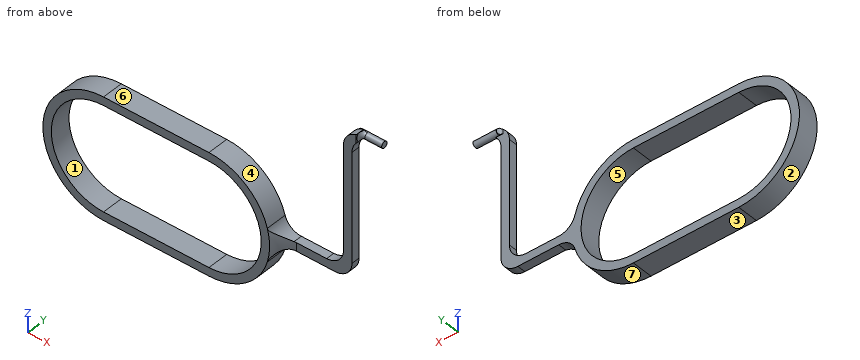
from build123d import *

# Parameters (mm, degrees)
BOSS_EXTRUDE1_DEPTH      = 5
BOSS_EXTRUDE2_START      = 2
SKETCH2_W                = 2
SKETCH2_H                = 2
SKETCH2_H_2              = 30.5
SKETCH2_W_2              = 1
BOSS_EXTRUDE2_DEPTH      = 2
FILLET1_R                = 4
BOSS_EXTRUDE3_DEPTH      = 5
BOSS_EXTRUDE3_DEPTH_BACK = 0.5
SKETCH3_R                = 0.75
FILLET2_R                = 1


with BuildPart() as part:
    # Sketch1 → Boss-Extrude1 (new body)
    with BuildSketch(Plane(origin=(0, 0, 0), x_dir=(1, 0, 0), z_dir=(0, 1, 0))):
        with BuildLine():
            Line((0, 14.4), (25, 14.4))
            ThreePointArc((25, 14.4), (39.4, 0), (25, -14.4))
            Line((25, -14.4), (0, -14.4))
            ThreePointArc((0, -14.4), (-14.4, 0), (0, 14.4))
        make_face()
        with BuildLine():
            Line((0, 12.4), (25, 12.4))
            ThreePointArc((25, 12.4), (37.4, 0), (25, -12.4))
            Line((25, -12.4), (0, -12.4))
            ThreePointArc((0, -12.4), (-12.4, 0), (0, 12.4))
        make_face(mode=Mode.SUBTRACT)
    extrude(amount=BOSS_EXTRUDE1_DEPTH)

    # Sketch2 → Boss-Extrude2 (add)
    with BuildSketch(Plane.XZ.offset(-5).offset(BOSS_EXTRUDE2_START)):
        with BuildLine():
            Line((39.365235814, -1), (54.4, -1))
            Line((54.4, -1), (54.4, 1))
            Line((54.4, 1), (39.365235814, 1))
            ThreePointArc((39.365235814, 1), (39.4, 0), (39.365235814, -1))
        make_face()
        with BuildLine():
            Line((37.4, -1), (39.365235814, -1))
            ThreePointArc((39.365235814, -1), (39.4, 0), (39.365235814, 1))
            Line((39.365235814, 1), (37.4, 1))
            Line((37.4, 1), (37.4, -1))
        make_face()
        with Locations((55.4, 0)):
            Rectangle(SKETCH2_W, SKETCH2_H)
        with Locations((55.4, 16.25)):
            Rectangle(SKETCH2_W, SKETCH2_H_2)
        with Locations((55.4, 32.5)):
            Rectangle(SKETCH2_W, SKETCH2_H)
        with Locations((56.9, 32.5)):
            Rectangle(SKETCH2_W_2, SKETCH2_H)
    extrude(amount=-BOSS_EXTRUDE2_DEPTH)

    # Fillet1
    # the kernel refuses this fillet: 4 mm, written as the material it adds along each edge
    with BuildSketch(Plane(origin=(25, 3, 0), x_dir=(0.7371891614816782, 0, -0.6756864214959037), z_dir=(-0.6756864214959037, 0, -0.7371891614816782))) as fillet1_piece_1_section:
        with BuildLine():
            CenterArc((18.272983346, 4), FILLET1_R, 194.477512186, 75.522487814)
            Line((18.272983346, 0), (18.272983346, -0.08))
            Line((18.272983346, -0.08), (14.4, -0.08))
            Line((14.4, -0.08), (14.32, 0))
            ThreePointArc((14.32, 0), (14.32, 1.5), (14.322540333, 2.98))
            Line((14.322540333, 2.98), (14.4, 3))
        make_face()
    fillet1_piece_1 = revolve(axis=Axis((25, 3, 0), (0, -1, 0)), revolution_arc=85.014954966, mode=Mode.PRIVATE)
    fillet1_piece_1 = split(fillet1_piece_1, bisect_by=Plane(origin=(40.301586348, 2.241602013, 1), z_dir=(0, 0, -1)), keep=Keep.TOP, mode=Mode.PRIVATE)
    fillet1_piece_1 = split(fillet1_piece_1, bisect_by=Plane(origin=(40.301586348, 2.241602013, -1), z_dir=(0, 0, 1)), keep=Keep.TOP, mode=Mode.PRIVATE)
    add(fillet1_piece_1)
    with BuildSketch(Plane(origin=(39.365235814, 5, 1), x_dir=(-0.17149804582148107, 0, 0.9851844600273663), z_dir=(0, -1, 0))) as fillet1_piece_2:
        with BuildLine():
            CenterArc((3.367524545, -3.978862537), FILLET1_R, 95.892851455, 74.232218513)
            Line((-0.573213295, -3.292870354), (-0.652028052, -3.27915051))
            Line((-0.652028052, -3.27915051), (-0.078814757, 0.013719844))
            Line((-0.078814757, 0.013719844), (0.008213474, 0.079577251))
            ThreePointArc((0.008213474, 0.079577251), (1.47842541, 0.003905135), (2.948637345, 0.079577251))
            Line((2.948637345, 0.079577251), (2.95685082, 0))
        make_face()
    extrude(amount=2)
    with BuildSketch(Plane(origin=(39.365235814, 5, -1), x_dir=(-0.17149804582148342, 0, -0.9851844600273658), z_dir=(0, -1, 0))) as fillet1_piece_3:
        with BuildLine():
            CenterArc((3.367524545, 3.978862537), FILLET1_R, 189.874930032, 74.232218513)
            Line((-0.573213295, 3.292870354), (-0.652028052, 3.27915051))
            Line((-0.652028052, 3.27915051), (-0.078814757, -0.013719844))
            Line((-0.078814757, -0.013719844), (0.008213474, -0.079577251))
            ThreePointArc((0.008213474, -0.079577251), (1.47842541, -0.003905135), (2.948637345, -0.079577251))
            Line((2.948637345, -0.079577251), (2.95685082, 0))
        make_face()
    extrude(amount=2)
    with BuildSketch(Plane(origin=(54.4, 3, 1), x_dir=(-1, 0, 0), z_dir=(0, 1, 0))) as fillet1_piece_4:
        with BuildLine():
            CenterArc((FILLET1_R, FILLET1_R), FILLET1_R, 180, 90)
            Line((0, FILLET1_R), (-FILLET1_R * 0.02, FILLET1_R))
            Line((-FILLET1_R * 0.02, FILLET1_R), (-FILLET1_R * 0.02, -FILLET1_R * 0.02))
            Line((-FILLET1_R * 0.02, -FILLET1_R * 0.02), (FILLET1_R, -FILLET1_R * 0.02))
            Line((FILLET1_R, -FILLET1_R * 0.02), (FILLET1_R, 0))
        make_face()
    extrude(amount=2)
    with BuildSketch(Plane(origin=(56.4, 3, 31.5), x_dir=(1, 0, 0), z_dir=(0, 1, 0))) as fillet1_piece_5:
        with BuildLine():
            CenterArc((4, 2.645751311), FILLET1_R, 180, 41.409622109)
            Line((0, 2.645751311), (-0.08, 2.645751311))
            Line((-0.08, 2.645751311), (-0.08, 0))
            Line((-0.08, 0), (0, -0.08))
            ThreePointArc((0, -0.08), (0.5, -0.08), (0.94, -0.052915026))
            Line((0.94, -0.052915026), (1, 0))
        make_face()
    extrude(amount=2)
    with BuildSketch(Plane(origin=(25, 3, 0), x_dir=(0.7371891614816782, 0, -0.6756864214959037), z_dir=(-0.6756864214959037, 0, -0.7371891614816782))) as fillet1_piece_6a_section:
        with BuildLine():
            CenterArc((18.272983346, 4), FILLET1_R, 194.477512186, 75.522487814)
            Line((18.272983346, 0), (18.272983346, -0.08))
            Line((18.272983346, -0.08), (14.4, -0.08))
            Line((14.4, -0.08), (14.32, 0))
            ThreePointArc((14.32, 0), (14.32, 1.5), (14.322540333, 2.98))
            Line((14.322540333, 2.98), (14.4, 3))
        make_face()
    fillet1_piece_6a = revolve(axis=Axis((25, 3, 0), (0, -1, 0)), revolution_arc=85.014954966, mode=Mode.PRIVATE)
    fillet1_piece_6a = split(fillet1_piece_6a, bisect_by=Plane(origin=(38.861424428, 2.266551756, -1), z_dir=(0, 0, -1)), keep=Keep.TOP, mode=Mode.PRIVATE)
    with BuildSketch(Plane(origin=(39.365235814, 5, -1), x_dir=(-0.17149804582148342, 0, -0.9851844600273658), z_dir=(0, -1, 0))) as fillet1_piece_6b_section:
        with BuildLine():
            CenterArc((3.367524545, 3.978862537), FILLET1_R, 189.874930032, 74.232218513)
            Line((-0.573213295, 3.292870354), (-0.652028052, 3.27915051))
            Line((-0.652028052, 3.27915051), (-0.078814757, -0.013719844))
            Line((-0.078814757, -0.013719844), (0.008213474, -0.079577251))
            ThreePointArc((0.008213474, -0.079577251), (1.47842541, -0.003905135), (2.948637345, -0.079577251))
            Line((2.948637345, -0.079577251), (2.95685082, 0))
        make_face()
    fillet1_piece_6b = extrude(amount=10.355974154, mode=Mode.PRIVATE)
    fillet1_piece_6b = split(fillet1_piece_6b, bisect_by=Plane(origin=(40.057221624, 0, -1.646357347), z_dir=(0, 1, 0)), keep=Keep.TOP, mode=Mode.PRIVATE)
    fillet1_piece_6b = split(fillet1_piece_6b, bisect_by=Plane(origin=(40.057221624, 3, -1.646357347), z_dir=(0, -1, 0)), keep=Keep.TOP, mode=Mode.PRIVATE)
    fillet1_piece_6 = fillet1_piece_6a & fillet1_piece_6b
    add(fillet1_piece_6)
    with BuildSketch(Plane(origin=(39.365235814, 5, 1), x_dir=(-0.17149804582148107, 0, 0.9851844600273663), z_dir=(0, -1, 0))) as fillet1_piece_7a_section:
        with BuildLine():
            CenterArc((3.367524545, -3.978862537), FILLET1_R, 95.892851455, 74.232218513)
            Line((-0.573213295, -3.292870354), (-0.652028052, -3.27915051))
            Line((-0.652028052, -3.27915051), (-0.078814757, 0.013719844))
            Line((-0.078814757, 0.013719844), (0.008213474, 0.079577251))
            ThreePointArc((0.008213474, 0.079577251), (1.47842541, 0.003905135), (2.948637345, 0.079577251))
            Line((2.948637345, 0.079577251), (2.95685082, 0))
        make_face()
    fillet1_piece_7a = extrude(amount=10.355974154, mode=Mode.PRIVATE)
    fillet1_piece_7a = split(fillet1_piece_7a, bisect_by=Plane(origin=(40.057221624, 0, 1.646357347), z_dir=(0, 1, 0)), keep=Keep.TOP, mode=Mode.PRIVATE)
    fillet1_piece_7a = split(fillet1_piece_7a, bisect_by=Plane(origin=(40.057221624, 3, 1.646357347), z_dir=(0, -1, 0)), keep=Keep.TOP, mode=Mode.PRIVATE)
    with BuildSketch(Plane(origin=(25, 3, 0), x_dir=(0.7371891614816782, 0, -0.6756864214959037), z_dir=(-0.6756864214959037, 0, -0.7371891614816782))) as fillet1_piece_7b_section:
        with BuildLine():
            CenterArc((18.272983346, 4), FILLET1_R, 194.477512186, 75.522487814)
            Line((18.272983346, 0), (18.272983346, -0.08))
            Line((18.272983346, -0.08), (14.4, -0.08))
            Line((14.4, -0.08), (14.32, 0))
            ThreePointArc((14.32, 0), (14.32, 1.5), (14.322540333, 2.98))
            Line((14.322540333, 2.98), (14.4, 3))
        make_face()
    fillet1_piece_7b = revolve(axis=Axis((25, 3, 0), (0, -1, 0)), revolution_arc=85.014954966, mode=Mode.PRIVATE)
    fillet1_piece_7b = split(fillet1_piece_7b, bisect_by=Plane(origin=(38.861423807, 2.266551545, 1), z_dir=(0, 0, 1)), keep=Keep.TOP, mode=Mode.PRIVATE)
    fillet1_piece_7 = fillet1_piece_7a & fillet1_piece_7b
    add(fillet1_piece_7)
    # the kernel refuses this fillet: 4 mm, written as the material it takes off along each edge
    with BuildSketch(Plane(origin=(56.4, -7, -1), x_dir=(0, 0, 1), z_dir=(0, 1, 0))) as fillet1_2_piece_1:
        with BuildLine():
            CenterArc((FILLET1_R, -FILLET1_R), FILLET1_R, 90, 90)
            Line((0, -FILLET1_R), (-FILLET1_R * 0.02, -FILLET1_R))
            Line((-FILLET1_R * 0.02, -FILLET1_R), (-FILLET1_R * 0.02, FILLET1_R * 0.02))
            Line((-FILLET1_R * 0.02, FILLET1_R * 0.02), (FILLET1_R, FILLET1_R * 0.02))
            Line((FILLET1_R, FILLET1_R * 0.02), (FILLET1_R, 0))
        make_face()
    extrude(amount=22, mode=Mode.SUBTRACT)
    with BuildSketch(Plane(origin=(54.4, -6.682458366, 33.5), x_dir=(0, 0, -1), z_dir=(0, 1, 0))) as fillet1_2_piece_2:
        with BuildLine():
            CenterArc((3.872983346, -4), FILLET1_R, 90, 75.522487814)
            Line((0, -3), (-0.077459667, -2.98))
            ThreePointArc((-0.077459667, -2.98), (-0.08, -1.5), (-0.08, 0))
            Line((-0.08, 0), (0, 0.08))
            Line((0, 0.08), (3.872983346, 0.08))
            Line((3.872983346, 0.08), (3.872983346, 0))
        make_face()
    extrude(amount=21.364916731, mode=Mode.SUBTRACT)

    # Sketch3 → Boss-Extrude3 (add, two sides: drawn at the far end of the back side and taken through both)
    with BuildSketch(Plane(origin=(57.4, 0, 0), x_dir=(0, 0, -1), z_dir=(1, 0, 0)).offset(-BOSS_EXTRUDE3_DEPTH_BACK)):
        with Locations((-32.5, 5)):
            Circle(SKETCH3_R)
    extrude(amount=BOSS_EXTRUDE3_DEPTH + BOSS_EXTRUDE3_DEPTH_BACK)

    # Fillet2
    # the kernel refuses this fillet: 1 mm, written as the material it adds along each edge
    with BuildSketch(Plane(origin=(56.9, 5, 29.25), x_dir=(-1, 0, 0), z_dir=(0, 0, 1))) as fillet2_piece_1_section:
        with BuildLine():
            CenterArc((FILLET2_R, -FILLET2_R), FILLET2_R, 90, 90)
            Line((0, -FILLET2_R), (0, 0))
            Line((0, 0), (FILLET2_R, 0))
        make_face()
    fillet2_piece_1 = extrude(amount=6.5, mode=Mode.PRIVATE)
    fillet2_piece_1 = fillet2_piece_1 & Plane(origin=(58.4, 5.187261993, 29.627016654), x_dir=(0, 0, -1), z_dir=(0, -1, 0)) * Cylinder(4, 17, mode=Mode.PRIVATE)
    fillet2_piece_1 = fillet2_piece_1 & Plane(origin=(56.665651888, 5, 32.5), x_dir=(0, 0, -1), z_dir=(1, 0, 0)) * Cylinder(0.75, 17, mode=Mode.PRIVATE)
    add(fillet2_piece_1)
    with BuildSketch(Plane(origin=(57.4, 5, 32.5), x_dir=(0, 0, 1), z_dir=(0, 1, 0))) as fillet2_piece_2_section:
        with BuildLine():
            CenterArc((0.75 + FILLET2_R, FILLET2_R), FILLET2_R, 180, 90)
            Line((0.75, FILLET2_R), (0.75, 0))
            Line((0.75, 0), (0.75 + FILLET2_R, 0))
        make_face()
    fillet2_piece_2 = revolve(axis=Axis((57.4, 5, 32.5), (1, 0, 0)), revolution_arc=180, mode=Mode.PRIVATE)
    fillet2_piece_2 = fillet2_piece_2 & Plane(origin=(58.4, 4.254671914, 29.627016654), x_dir=(0, 0, -1), z_dir=(0, -1, 0)) * Cylinder(4, 7, mode=Mode.PRIVATE)
    fillet2_piece_2 = fillet2_piece_2 - Plane(origin=(60.4, 4.254671914, 28.854248689), x_dir=(1, 0, 0), z_dir=(0, -1, 0)) * Cylinder(4, 7, mode=Mode.PRIVATE)
    add(fillet2_piece_2)


solid = part.part
Build history of the part. All positions in model axes, mm. Face numbers are marked on the shaded views. A direction names the side the tool comes from. Coordinates: 2 decimals unless noted, no trailing zeros. Order: outer loops, then holes, each group sorted by start corner. A loop starts at its lowest first (then second) coordinate and runs counter-clockwise, first axis right, second up. Notation, with made-up numbers: (41.5, 53) -> (67.5, 53) arc R28 cw to (67.5, 75) -> close; hole circle Ø7 at (-0.75, 43.25). An arc over 180 degrees is marked (long way). One line per item, written item: value.
(1) Slice it at B-B, the plane y = 1.45. List the corners of the cut face in (x, z), plus the area to 3 significant figures.
Checked values:
outline: (0, -14.4) -> (25, -14.4) arc R14.4 ccw to (38.86, -3.91) arc R4 cw to (39.97, -2.09) arc R15.11 ccw to (39.97, 2.09) arc R4 cw to (38.86, 3.91) arc R14.4 ccw to (25, 14.4) -> (0, 14.4) arc R14.4 ccw to start; hole (0, -12.4) -> (25, -12.4) arc R12.4 ccw to (25, 12.4) -> (0, 12.4) arc R12.4 ccw to start
area: 272 mm2
(2) Slice it at C-C, the plane z = -8. List the corners of the cut face in (x, y).
Checked values:
outline: (-11.97, 0) -> (-9.47, 0) -> (-9.47, 5) -> (-11.97, 5) -> close; (34.47, 0) -> (36.97, 0) -> (36.97, 5) -> (34.47, 5) -> close
(3) Tool access for the marked faces 5, 6 and 7: list every direction of +Z, -Z, +X, -X, +Y, -Y with a clear straight run to the whole face (end or side of a thin tool).
Checked values:
face 5: +Y, -Y
face 6: +Z, -X, +Y, -Y
face 7: -Z, +X, +Y, -Y
(4) Mould opens along X. For the marked faces 1, 2, 3 and 4 say: pulls with the +X half, pulls with the -X half, needs draft (parallel to the pull), parting line crosses it, or undercut.
Checked values:
face 1: undercut
face 2: pulls with the -X half
face 3: needs draft
face 4: undercut
(5) Drop flat-ended pins along their axis: pin 1 Ø1.6 at (y, z) = (4, 13) entering from -X; pin 2 Ø1.6 at (y, z) = (4, 18.5) entering from +X; pin 3 Ø1.6 at (x, y) = (46, 3.5) entering from -Z. Give the stop position or say it passes through.
Checked values:
pin 1: x = -7.65
pin 2: x = 56.4
pin 3: z = -1
(6) Probe line 1 (Z direction, x = 22, y = 2.2); line 2 (X direction, y = 4.9, z = 1.5); line 3 (X direction, y = 4.5, z = 2). List the from-to ranges inside material, lowest first. Write a range as [from, to].
Checked values:
line 1: [-14.4, -12.4], [12.4, 14.4]
line 2: [-14.32, -12.31], [37.31, 40.77], [52.34, 56.11]
line 3: [-14.26, -12.24], [37.24, 40.06], [53.05, 56.27]
(7) Slice it at A-A, the plane x = 22.5. List the corners of the cut face in (y, z), plus the area to 3 significant figures.
Checked values:
outline: (0, -14.4) -> (5, -14.4) -> (5, -12.4) -> (0, -12.4) -> close; (0, 12.4) -> (5, 12.4) -> (5, 14.4) -> (0, 14.4) -> close
area: 20.0 mm2
(8) Slice it at D-D, the plane z = 25.5. List the corners of the cut face in (x, y), plus the area to 3 significant figures.
Checked values:
outline: (54.4, 3) -> (56.4, 3) -> (56.4, 5) -> (54.4, 5) -> close
area: 4.00 mm2
